Verification items for the finished model (mm, model axes). Give positions to 0.01 mm unless a question says otherwise; leave off trailing zeros. Write each loop counter-clockwise with the first axis right and the second up, starting at its lowest first coordinate (ties: lowest second). Pieces come first, ordered by that corner, then holes. Notation, with made-up numbers: (40.25, 82.25) - (90.25, 82.25) arc R22 ccw to (90.25, 92.25) - close; hole circle Ø4 at (71, 64.5). An arc over 180 degrees is marked (long way). Answer as a JSON object with one key per item and string values. Group by question number.
Item 1: Sectioned sample at A-A, the plane x = 4.25. Record the boundary of the cut face in (y, z), and give its area (4 significant figures).
Item 2: Scan lines: line 1 along X through (y, z) = (115, -3.9); line 2 along Y through (x, z) = (4.25, -2.9); line 3 along Y through (x, z) = (-6, -2.8). Record each from-to range of solid material in increasing order. Write a range as [from, to].
Item 3: Go/stop test with flat-tipped pins: pin 1 (1.5 mm diameter, centred on x = 0, y = 115, fed in from +Z); pin 2 (2 mm diameter, centred on x = 8, z = -2.5, fed in from +Y). Record where each tip stops, or that it passes through.
```python
from build123d import *

# Parameters (mm, degrees)
AUFSATZ_LINEAR_AUSTRAGEN1_DEPTH      = 12.5
AUFSATZ_LINEAR_AUSTRAGEN1_DEPTH_BACK = 12.5
SKIZZE1_W                            = 5
SKIZZE1_H                            = 175
M3_GEWINDEBOHRUNG3_D                 = 2.5
M3_GEWINDEBOHRUNG1_D                 = 2.5
M3_GEWINDEBOHRUNG1_DEPTH             = 8.5
M3_GEWINDEBOHRUNG1_TIP               = 0.751075774
M3_GEWINDEBOHRUNG2_D                 = 2.5
M3_GEWINDEBOHRUNG2_DEPTH             = 8.5
M3_GEWINDEBOHRUNG2_TIP               = 0.751075774
DURCHGANGSLOCH_F_R_M41_D             = 4.3


with BuildPart() as part:
    # Skizze1 → Aufsatz-Linear austragen1 (new, two sides: drawn at the far end of the back side and taken through both)
    with BuildSketch(Plane(origin=(0, 0, 0), x_dir=(0, 0, -1), z_dir=(1, 0, 0)).offset(-AUFSATZ_LINEAR_AUSTRAGEN1_DEPTH_BACK)):
        with Locations((2.5, 87.5)):
            Rectangle(SKIZZE1_W, SKIZZE1_H)
    extrude(amount=AUFSATZ_LINEAR_AUSTRAGEN1_DEPTH + AUFSATZ_LINEAR_AUSTRAGEN1_DEPTH_BACK)

    # M3 Gewindebohrung3 (through all)
    with Locations(Plane(origin=(0, 0, -5), x_dir=(-1, 0, 0), z_dir=(0, 0, -1))):
        with Locations((0, 15), (0, 165), (0, 140), (0, 115), (0, 90), (0, 65), (0, 40)):
            Hole(M3_GEWINDEBOHRUNG3_D / 2)

    # M3 Gewindebohrung1
    with Locations(Plane(origin=(0, 175, 0), x_dir=(1, 0, 0), z_dir=(0, 1, 0))):
        with Locations((8, 2.5), (-8, 2.5)):
            Hole(M3_GEWINDEBOHRUNG1_D / 2, depth=M3_GEWINDEBOHRUNG1_DEPTH)
            with Locations((0, 0, -(M3_GEWINDEBOHRUNG1_DEPTH + M3_GEWINDEBOHRUNG1_TIP / 2))):  # 118° drill point
                Cone(0, M3_GEWINDEBOHRUNG1_D / 2, M3_GEWINDEBOHRUNG1_TIP, mode=Mode.SUBTRACT)

    # M3 Gewindebohrung2
    with Locations(Plane(origin=(0, 0, 0), x_dir=(-1, 0, 0), z_dir=(0, -1, 0))):
        with Locations((8, 2.5), (-8, 2.5)):
            Hole(M3_GEWINDEBOHRUNG2_D / 2, depth=M3_GEWINDEBOHRUNG2_DEPTH)
            with Locations((0, 0, -(M3_GEWINDEBOHRUNG2_DEPTH + M3_GEWINDEBOHRUNG2_TIP / 2))):  # 118° drill point
                Cone(0, M3_GEWINDEBOHRUNG2_D / 2, M3_GEWINDEBOHRUNG2_TIP, mode=Mode.SUBTRACT)

    # Durchgangsloch für M41 (through all)
    with Locations(Plane(origin=(0, 0, -5), x_dir=(-1, 0, 0), z_dir=(0, 0, -1))):
        with Locations((-4.25, 8), (4.25, 8)):
            Hole(DURCHGANGSLOCH_F_R_M41_D / 2)


solid = part.part
```
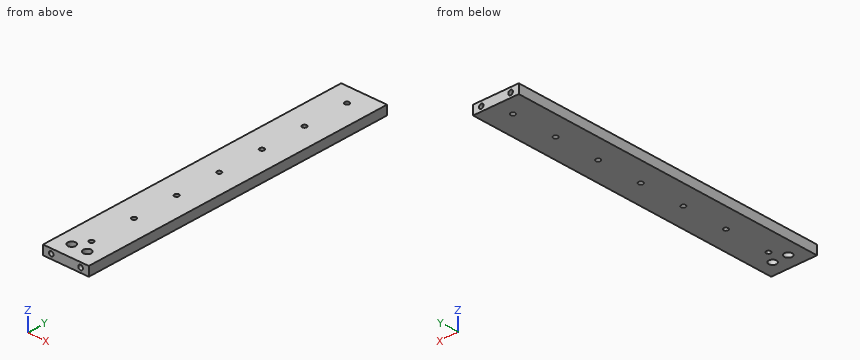
Geometry check:
{
 "1": {"outline": "(0, -5) - (5.85, -5) - (5.85, 0) - (0, 0) - close; (10.15, -5) - (175, -5) - (175, 0) - (10.15, 0) - close", "area": "853.5 mm^2"},
 "2": {"line 1": "[-12.5, -1.25], [1.25, 12.5]", "line 2": "[0, 5.85], [10.15, 175]", "line 3": "[0, 6.75], [9.25, 175]"},
 "3": {"pin 1": "through", "pin 2": "y = 166.35"}
}
